```python
from build123d import *

# Parameters (mm, degrees)
ESQUISSE1_R             = 13
ESQUISSE1_R_2           = 2.75
ESQUISSE1_R_3           = 1.65
BOSS_EXTRU_1_DEPTH      = 10
ESQUISSE2_R             = 10.5
ENL_V_MAT_EXTRU_1_DEPTH = 3
ESQUISSE3_R             = 2.75
ENL_V_MAT_EXTRU_2_DEPTH = 5.5
ESQUISSE4_R             = 1
BOSS_EXTRU_2_DEPTH      = 3


with BuildPart() as part:
    # Esquisse1 → Boss.-Extru.1 (new body)
    with BuildSketch(Plane.XY):
        Circle(ESQUISSE1_R)
        Circle(ESQUISSE1_R_2, mode=Mode.SUBTRACT)
        with Locations((-7, 0)):
            Circle(ESQUISSE1_R_3, mode=Mode.SUBTRACT)
        with Locations((0, 7)):
            Circle(ESQUISSE1_R_3, mode=Mode.SUBTRACT)
        with Locations((7, 0)):
            Circle(ESQUISSE1_R_3, mode=Mode.SUBTRACT)
        with Locations((0, -7)):
            Circle(ESQUISSE1_R_3, mode=Mode.SUBTRACT)
    extrude(amount=BOSS_EXTRU_1_DEPTH)

    # Esquisse2 → Enlèv. mat.-Extru.1 (cut)
    with BuildSketch(Plane.XY.offset(10)):
        Circle(ESQUISSE2_R)
    extrude(amount=-ENL_V_MAT_EXTRU_1_DEPTH, mode=Mode.SUBTRACT)

    # Esquisse3 → Enlèv. mat.-Extru.2 (cut)
    with BuildSketch(Plane(origin=(0, 0, 0), x_dir=(-1, 0, 0), z_dir=(0, 0, -1))):
        with Locations((-7, 0)):
            Circle(ESQUISSE3_R)
        with Locations((0, 7)):
            Circle(ESQUISSE3_R)
        with Locations((7, 0)):
            Circle(ESQUISSE3_R)
        with Locations((0, -7)):
            Circle(ESQUISSE3_R)
    extrude(amount=-ENL_V_MAT_EXTRU_2_DEPTH, mode=Mode.SUBTRACT)

    # Esquisse4 → Boss.-Extru.2 (add)
    with BuildSketch(Plane(origin=(0, 0, 0), x_dir=(-1, 0, 0), z_dir=(0, 0, -1))):
        with BuildLine():
            Line((-4, 28.369316877), (-4, 12.369316877))
            ThreePointArc((-4, 12.369316877), (0, 13), (4, 12.369316877))
            Line((4, 12.369316877), (4, 28.369316877))
            ThreePointArc((4, 28.369316877), (0, 32.369316877), (-4, 28.369316877))
        make_face()
        with Locations((0, 28.369316877)):
            Circle(ESQUISSE4_R, mode=Mode.SUBTRACT)
    boss_extru_2 = extrude(amount=-BOSS_EXTRU_2_DEPTH)

    # Symétrie1: Boss.-Extru.2 across plane
    add(boss_extru_2.mirror(Plane.XY.offset(5)))


solid = part.part
```
Can you work these out from the model? Positions are in its coordinate system, mm. A direction names the side the tool comes from. Coordinates: 2 decimals unless noted, no trailing zeros. Order: outer loops, then holes, each group sorted by start corner. A loop starts at its lowest first (then second) coordinate and runs counter-clockwise, first axis right, second up. Notation, with made-up numbers: (46, 46) -> (54, 46) arc R13 ccw to (54, 65) -> close; hole circle Ø4 at (-26, 6). An arc over 180 degrees is marked (long way). Write each question's results on one line, items separated by ' | '.
Item 1: Which directions (+Z, -Z, +X, -X, +Y, -Y) give clear straight access to the entire face, cutting with the end or side of a thin tool? Please do faces 4 (the face through (4, 20, 1)), 5 (the face through (-0.09, 32.37, 8.52)), 6 (the face through (-4, 20, 9)), 7 (the face through (10, 3.2, 8.5)), 8 (the face through (0, -9, 5.5)).
Results are:
face 4: +Z, -Z, +X, +Y | face 5: +Z, -Z, +Y | face 6: +Z, -Z, -X, +Y | face 7: +Z | face 8: -Z
Item 2: I want a section at C-C, the plane z = 8.25. Write out the boundary of the cut face in (x, y).
Results are:
outline: (-4, 12.37) arc R13 ccw (long way) to (4, 12.37) -> (4, 28.37) arc R4 ccw to (-4, 28.37) -> close; hole circle Ø21 at (0, 0); hole circle Ø2 at (0, 28.37)
Item 3: If I drill on line 1 along Y through (x, z) = (0, 5.9); line 2 along Y through (x, z) = (0, 1.55); line 3 along Y through (x, z) = (0, 4.2), over which ranges is the centre line in solid material (lowest first)?
Results are:
line 1: -13 to -8.65, -5.35 to -2.75, 2.75 to 5.35, 8.65 to 13 | line 2: -13 to -9.75, -4.25 to -2.75, 2.75 to 4.25, 9.75 to 27.37, 29.37 to 32.37 | line 3: -13 to -9.75, -4.25 to -2.75, 2.75 to 4.25, 9.75 to 13
Item 4: I want a section at A-A, the plane y = 0. Write out the boundary of the cut face in (x, z), then the cut area to 3 significant figures.
Results are:
outline: (-13, 0) -> (-9.75, 0) -> (-9.75, 5.5) -> (-8.65, 5.5) -> (-8.65, 7) -> (-10.5, 7) -> (-10.5, 10) -> (-13, 10) -> close; (-5.35, 5.5) -> (-4.25, 5.5) -> (-4.25, 0) -> (-2.75, 0) -> (-2.75, 7) -> (-5.35, 7) -> close; (2.75, 0) -> (4.25, 0) -> (4.25, 5.5) -> (5.35, 5.5) -> (5.35, 7) -> (2.75, 7) -> close; (8.65, 5.5) -> (9.75, 5.5) -> (9.75, 0) -> (13, 0) -> (13, 10) -> (10.5, 10) -> (10.5, 7) -> (8.65, 7) -> close | area: 88.1 mm²
Item 5: I'm going to push flat-ended pins straight in: pin 1 Ø6 at (x, y) = (1.5, 7) entering from -Z; pin 2 Ø2 at (y, z) = (22, 6.5) entering from +X; pin 3 Ø4 at (x, y) = (0, 7) entering from -Z; pin 4 Ø3.5 at (y, z) = (18, 8.5) entering from -X. Where does each tip first touch, or does it pass through?
Results are:
pin 1: z = 0 | pin 2: x = 4 | pin 3: z = 5.5 | pin 4: x = -4
Item 6: I want a section at B-B, the plane x = -7. Write out the boundary of the cut face in (y, z), then the cut area to 3 significant figures.
Results are:
outline: (-10.95, 0) -> (-2.75, 0) -> (-2.75, 5.5) -> (-1.65, 5.5) -> (-1.65, 7) -> (-7.83, 7) -> (-7.83, 10) -> (-10.95, 10) -> close; (1.65, 5.5) -> (2.75, 5.5) -> (2.75, 0) -> (10.95, 0) -> (10.95, 10) -> (7.83, 10) -> (7.83, 7) -> (1.65, 7) -> close | area: 137 mm²
Item 7: If we mould it in two halves opening along X, with no side actions, what happens to faces 1 (the face through (5, 0, 5.5)), 2 (the face through (1, 11, 10)), 3 (the face through (-4, 20, 1))? For each: +X half, -X half, draft (parallel to the pull), parting line (faces both ways), or undercut.
Results are:
face 1: undercut | face 2: draft | face 3: -X half
Item 8: I want a section at D-D, the plane y = 22. Write out the boundary of the cut face in (x, z), then the cut area to 3 significant figures.
Results are:
outline: (-4, 0) -> (4, 0) -> (4, 3) -> (-4, 3) -> close; (-4, 7) -> (4, 7) -> (4, 10) -> (-4, 10) -> close | area: 48.0 mm²
